Could you check a few things on this model? Use its own coordinates, in mm. Face numbers are marked on the shaded views. A direction names the side the tool comes from. Coordinates: 2 decimals unless noted, no trailing zeros. Loops run counter-clockwise (first coordinate to the right, second up) from the corner with the lowest first, then second, coordinate; pieces in that order, holes last. Notation, with made-up numbers: M -9.75,72 L 12.25,72 A10 cw 12.25,90 Z; hole C -30,-31.5 d7. An arc over 180 degrees is marked long. Write each question's results on one line, items separated by ' | '.
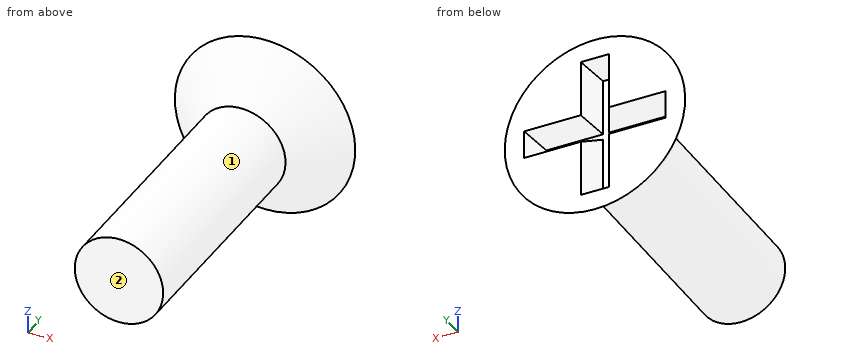
```python
from build123d import *

# Parameters (mm, degrees)
CUT_EXTRUDE_1_DEPTH = 0.6
CUT_EXTRUDE_1_DRAFT = -28


with BuildPart() as part:
    # Эскиз1 → Повернуть1 (revolve)
    with BuildSketch(Plane.XY, mode=Mode.PRIVATE) as revolve_1_sk:
        Polygon((0, 8), (-2.55, 8), (-1.25, 6.7), (-1.25, 0), (0, 0), align=None)
    revolve(revolve_1_sk.sketch.rotate(Axis((0, 0, 0), (0, 1, 0)), 270), axis=Axis((0, 0, 0), (0, 1, 0)))


with BuildPart() as cut_extrude_1_tool:
    # Эскиз2 → Вырез-Вытянуть1 (with draft: the straight prism first)
    with BuildSketch(Plane(origin=(0, 8, 0), x_dir=(1, 0, 0), z_dir=(0, 1, 0))):
        Polygon((0.4, 0.4), (0.4, 2), (-0.4, 2), (-0.4, 0.4), (-2, 0.4), (-2, -0.4), (-0.4, -0.4), (-0.4, -2), (0.4, -2), (0.4, -0.4), (2, -0.4), (2, 0.4), align=None)
    extrude(amount=-CUT_EXTRUDE_1_DEPTH)
    # Вырез-Вытянуть1: the draft: its side faces are tilted about the plane it starts from
    cut_extrude_1_sides = [cut_extrude_1_tool.faces().sort_by_distance(p)[0] for p in [
        (0.4, 7.7, -1.2),
        (0, 7.7, -2),
        (-0.4, 7.7, -1.2),
        (-1.2, 7.7, -0.4),
        (-2, 7.7, 0),
        (-1.2, 7.7, 0.4),
        (-0.4, 7.7, 1.2),
        (0, 7.7, 2),
        (0.4, 7.7, 1.2),
        (1.2, 7.7, 0.4),
        (2, 7.7, 0),
        (1.2, 7.7, -0.4),
    ]]
    draft(cut_extrude_1_sides, Plane(origin=(0, 8, 0), x_dir=(1, 0, 0), z_dir=(0, 1, 0)), CUT_EXTRUDE_1_DRAFT)


with BuildPart() as part_1:
    add(part.part)

    # Вырез-Вытянуть1: cut by cut_extrude_1_tool
    add(cut_extrude_1_tool.part, mode=Mode.SUBTRACT)


solid = part_1.part
```
(1) Imagine slicing it at B-B, the plane y = 5. List the corners of the cut face in (x, z) for me.
Reported:
outline: C 0,0 d2.5
(2) Imagine slicing it at A-A, the plane y = 7.25. List the corners of the cut face in (x, z) for me, and give its area (3 significant figures).
Reported:
outline: C 0,0 d3.6 | area: 10.2 mm2
(3) Which directions (+Z, -Z, +X, -X, +Y, -Y) give clear straight access to the entire face, cutting with the end or side of a thin tool? Please do the marked faces 1 and 2.
Reported:
face 1: -Y | face 2: +Z, -Z, +X, -X, -Y
(4) Please list where these lines run through material, in increasing order: probe 1 along Z at (x, y) = (-0.7, 3); probe 2 along X at (y, z) = (6.25, 0.1); probe 3 along Z at (x, y) = (0.6, 6). Write a range as from..to.
Reported:
probe 1: z = -1.04..1.04 | probe 2: x = -1.25..1.25 | probe 3: z = -1.1..1.1
(5) Will these pins go through, and if not, where does the flat tip stop? P1, Ø1.5, axis at y = 5, z = -0.5, coming from the -X side; P2, Ø1.5, axis at y = 7, z = -1.5, coming from the -X side; P3, Ø2, axis at x = 2, y = 5.5, coming from the -Z side.
Reported:
P1: stops at x = -1.25 | P2: stops at x = -1.89 | P3: stops at z = -0.75
